Verification items for the finished model (mm, model axes). Coordinates: 2 decimals unless noted, no trailing zeros. Order: outer loops, then holes, each group sorted by start corner. A loop starts at its lowest first (then second) coordinate and runs counter-clockwise, first axis right, second up.
Q1. Cross-section at A-A, the plane x = 60.9. Record the boundary of the cut face in (y, z).
Q2. Thickness scan on line 1 (X direction, y = 1.1, z = -4.5); line 2 (Z direction, x = 34, y = 2.45); line 3 (X direction, y = 0.2, z = 30). Record the ranges inside material, lowest first.
Q3. Cross-section at B-B, the plane x = -52.5. Record the boundary of the cut face in (y, z).
Q4. Draft check along Z on faces 1 (the flat face through (-33, 3, 29)), 2 (the cylindrical face through (-87.39, 1.48, -69.4)). Enter one of: pulls with the +Z half, pulls with the -Z half, needs draft (parallel to the pull), parting line crosses it, or undercut.
Q5. Depth check by flat-ended pin: P1, Ø1.5, axis at x = 39, y = 1.5, coming from the -Z side; P2, Ø0.9, axis at y = 1, z = 73.5, coming from the +X side; P3, Ø12, axis at x = 40.5, z = 11, coming from the +Y side. Enter the tip coordinate at first touch or a pass-through.
Q6. Cross-section at C-C, the plane y = 0.75. Count the separate pieces of the cut face and the enclosed holes in it, and give its area (3 significant figures).
Q7. Cross-section at D-D, the plane x = -72.5. Record the boundary of the cut face in (y, z).
from build123d import *

# Parameters (mm, degrees)
SKETCH1_R           = 2.5
SKETCH1_W           = 39.504270757
SKETCH1_H           = 34.26660973
BOSS_EXTRUDE1_DEPTH = 3
SKETCH4_R           = 2
CUT_EXTRUDE3_DEPTH  = 10


with BuildPart() as part:
    # Sketch1 → Boss-Extrude1 (new body)
    with BuildSketch(Plane(origin=(0, 0, 0), x_dir=(1, 0, 0), z_dir=(0, 1, 0))):
        Polygon((-100, 76.642236505), (-100, -98.157625791), (3, -98.157625791), (3, -45.195936932), (75.604056887, -45.195936932), (75.604056887, 12.636866249), (-0.5895682, 12.636866249), (-21.164811555, 12.447038184), (-21.164811555, -18.271243478), (-67.980697631, -18.271243478), (-67.980697631, 12.636866249), (-67.980697631, 76.642236505), align=None)
        with Locations(Location((-52.5, -70.657625791, 0), (0, 0, 270))):
            Circle(SKETCH1_R, mode=Mode.SUBTRACT)
        with Locations(Location((-72.5, -50.657625791, 0), (0, 0, 270))):
            Circle(SKETCH1_R, mode=Mode.SUBTRACT)
        with Locations(Location((-52.5, -30.657625791, 0), (0, 0, 270))):
            Circle(SKETCH1_R, mode=Mode.SUBTRACT)
        with Locations(Location((-32.5, -50.657625791, 0), (0, 0, 270))):
            Circle(SKETCH1_R, mode=Mode.SUBTRACT)
        with Locations(Location((-5, -13.657625791, 0), (0, 0, 270))):
            Circle(SKETCH1_R, mode=Mode.SUBTRACT)
        with Locations(Location((60.9, -13.657625791, 0), (0, 0, 270))):
            Circle(SKETCH1_R, mode=Mode.SUBTRACT)
        with Locations(Location((-89.5, -3.157625791, 0), (0, 0, 270))):
            Circle(SKETCH1_R, mode=Mode.SUBTRACT)
        with Locations(Location((-89.5, 62.742374209, 0), (0, 0, 270))):
            Circle(SKETCH1_R, mode=Mode.SUBTRACT)
        with Locations(Location((-89.5, 4.842374209, 0), (0, 0, 270))):
            Circle(SKETCH1_R, mode=Mode.SUBTRACT)
        with Locations(Location((-89.5, 70.742374209, 0), (0, 0, 270))):
            Circle(SKETCH1_R, mode=Mode.SUBTRACT)
        with Locations(Location((3, -13.657625791, 0), (0, 0, 270))):
            Circle(SKETCH1_R, mode=Mode.SUBTRACT)
        with Locations(Location((68.9, -13.657625791, 0), (0, 0, 270))):
            Circle(SKETCH1_R, mode=Mode.SUBTRACT)
        with Locations((32.721465803, -15.366695135)):
            Rectangle(SKETCH1_W, SKETCH1_H, mode=Mode.SUBTRACT)
    extrude(amount=BOSS_EXTRUDE1_DEPTH)

    # Sketch4 → Cut-Extrude3 (cut)
    with BuildSketch(Plane(origin=(0, 3, 0), x_dir=(1, 0, 0), z_dir=(0, 1, 0))):
        with Locations((-63.221437818, -7.837794837)):
            Circle(SKETCH4_R)
        with Locations((-26.595771041, -7.837794837)):
            Circle(SKETCH4_R)
        with Locations(Location((-89.563443469, -89.007054179, 0), (0, 0, 270))):
            Circle(SKETCH4_R)
        with Locations(Location((-10.164633565, -89.007054179, 0), (0, 0, 270))):
            Circle(SKETCH4_R)
        with Locations(Location((-10.164633565, -39.007054179, 0), (0, 0, 270))):
            Circle(SKETCH4_R)
        with Locations(Location((-89.563443469, -39.007054179, 0), (0, 0, 270))):
            Circle(SKETCH4_R)
    extrude(amount=-CUT_EXTRUDE3_DEPTH, mode=Mode.SUBTRACT)


solid = part.part
Check values:
1. outline: (0, -12.64) - (3, -12.64) - (3, 11.16) - (0, 11.16) - close; (0, 16.16) - (3, 16.16) - (3, 45.2) - (0, 45.2) - close
2. line 1: x = -100 to -91.98, -87.02 to -67.98, -21.16 to 75.6
2. line 2: z = -12.64 to -1.77, 32.5 to 45.2
2. line 3: x = -100 to -54.91, -50.09 to 12.97, 52.47 to 75.6
3. outline: (0, 18.27) - (3, 18.27) - (3, 28.16) - (0, 28.16) - close; (0, 33.16) - (3, 33.16) - (3, 68.16) - (0, 68.16) - close; (0, 73.16) - (3, 73.16) - (3, 98.16) - (0, 98.16) - close
4. face 1: needs draft
4. face 2: undercut
5. P1: stops at z = -12.64
5. P2: stops at x = 3
5. P3: passes through
6. separate pieces: 1
6. enclosed holes: 17
6. area: 14,600 mm2
7. outline: (0, -76.64) - (3, -76.64) - (3, 48.16) - (0, 48.16) - close; (0, 53.16) - (3, 53.16) - (3, 98.16) - (0, 98.16) - close
